from build123d import *

# Parameters (mm, degrees)
IZIM2_R               = 2
KES_EKSTR_ZYON1_DEPTH = 10
RADYUS1_R             = 0.4


with BuildPart() as part:
    # Çizim1 → Döndür1 (revolve)
    with BuildSketch(Plane.XY, mode=Mode.PRIVATE) as d_nd_r1_sk:
        Polygon((0, 0), (0, 35.4), (2, 35.4), (2, 20), (2.5, 20), (2.5, 0), align=None)
    revolve(d_nd_r1_sk.sketch.rotate(Axis((0, 0, 0), (0, 1, 0)), 90), axis=Axis((0, 0, 0), (0, 1, 0)))

    # Çizim2 → Kes-Ekstrüzyon1 (cut)
    with BuildSketch(Plane.XZ):
        with Locations(Location((0, 0, 0), (0, 0, 270))):
            Circle(IZIM2_R)
    extrude(amount=-KES_EKSTR_ZYON1_DEPTH, mode=Mode.SUBTRACT)

    # Radyus1
    radyus1_edges = [part.edges().sort_by_distance(p)[0] for p in [
        (0, 0, 2),
    ]]
    fillet(radyus1_edges, radius=RADYUS1_R)


solid = part.part
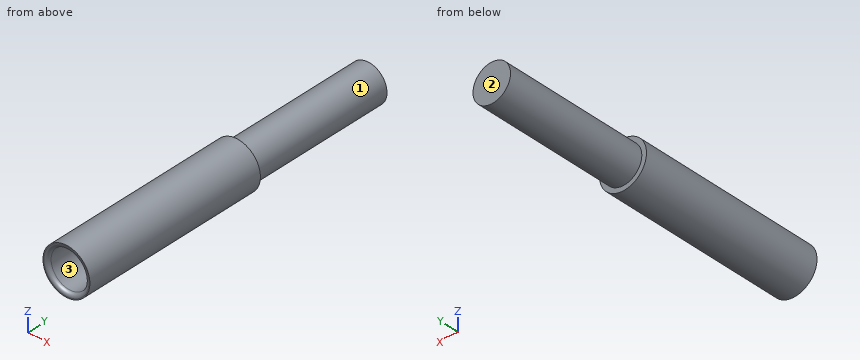
The model under review builds one solid part; all positions refer to its coordinate system, in mm. Face numbers are marked on the shaded views. Round coordinates to 2 decimals unless told otherwise and drop trailing zeros. Order: outer loops, then holes, each group sorted by start corner. A loop starts at its lowest first (then second) coordinate and runs counter-clockwise, first axis right, second up. Notation, with made-up numbers: (88.5, 17) - (101.5, 17) arc R18 cw to (101.5, 21) - close; hole circle Ø11 at (-36.75, -5.5). An arc over 180 degrees is marked (long way). Use one line per item in the form item = value.
Q1. Add section B-B on y = 8.5. Give the boundary of the cut face in (x, z).
Response values:
outline = circle Ø5 at (0, 0); hole circle Ø4 at (0, 0)
Q2. Mouldability with a two-part tool opening along X and no side actions: class the marked faces 1, 2 and 3 as pulls with the +X half, pulls with the -X half, needs draft (parallel to the pull), parting line crosses it, or undercut.
Response values:
face_1 = parting line crosses it
face_2 = needs draft
face_3 = undercut
Q3. To check wall thickness, follow line 1 (X direction, y = 3.5, z = 0); line 2 (Y direction, x = 1.2, z = -0.35); line 3 (Z direction, x = 0.8, y = 2). State the ranges of each line that lie inside material, in increasing order.
Response values:
line_1 = -2.5 to -2, 2 to 2.5
line_2 = 10 to 35.4
line_3 = -2.37 to -1.83, 1.83 to 2.37
Q4. Add section A-A on x = 0. Give the boundary of the cut face in (y, z), then the cut area to 3 significant figures.
Response values:
outline = (0, -2.5) - (20, -2.5) - (20, -2) - (35.4, -2) - (35.4, 2) - (20, 2) - (20, 2.5) - (0, 2.5) - (0, 2.4) arc R0.4 ccw to (0.4, 2) - (10, 2) - (10, -2) - (0.4, -2) arc R0.4 ccw to (0, -2.4) - close
area = 122 mm^2
Q5. Clearance check with flat-ended pins moving along their axes: P1, Ø1.5, axis at y = 15.5, z = 2, coming from the +X side; P2, Ø1.2, axis at x = 1, z = 0, coming from the -Y side; P3, Ø2, axis at y = 6, z = 1.5, coming from the +X side. State where each tip first meets the part, or that it passes through.
Response values:
P1 = 2.17
P2 = 10
P3 = 2.45
Q6. Add section C-C on z = 0. Give the boundary of the cut face in (x, y).
Response values:
outline = (-2.5, 0) - (-2.4, 0) arc R0.4 ccw to (-2, 0.4) - (-2, 10) - (2, 10) - (2, 0.4) arc R0.4 ccw to (2.4, 0) - (2.5, 0) - (2.5, 20) - (2, 20) - (2, 35.4) - (-2, 35.4) - (-2, 20) - (-2.5, 20) - close
Q7. Add section D-D on y = 30. Give the boundary of the cut face in (x, z).
Response values:
outline = circle Ø4 at (0, 0)
